Work out the finished part from the listing and answer in its coordinate system (mm). Give positions to 0.01 mm unless a question says otherwise; leave off trailing zeros. Loops run counter-clockwise (first coordinate to the right, second up) from the corner with the lowest first, then second, coordinate; pieces in that order, holes last. Notation, with made-up numbers: M 29.5,35 L 75.5,35 A7 ccw 75.5,40 Z; hole C 15.25,-0.75 d6. An arc over 180 degrees is marked long. Answer in a Markdown table with one row per item. Add a question column.
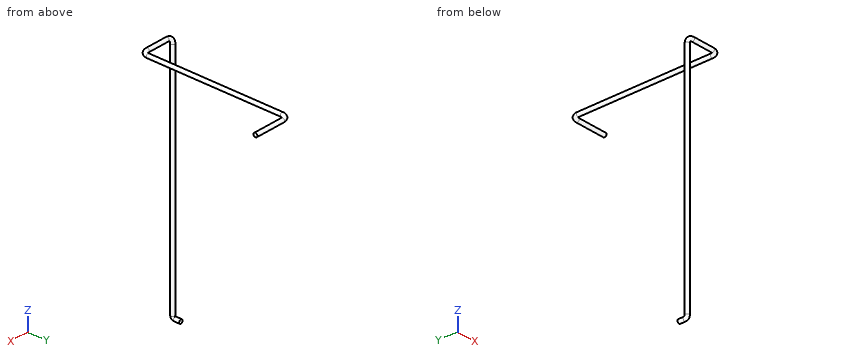
from build123d import *

# Parameters (mm, degrees)
CROQUIS1_R              = 9.525
SALIENTE_EXTRUIR1_DEPTH = 10
CROQUIS2_R              = 9.525


with BuildPart() as part:
    # Croquis1 → Saliente-Extruir1 (new body)
    with BuildSketch(Plane(origin=(0, 0, 0), x_dir=(1, 0, 0), z_dir=(0, 1, 0))):
        with Locations(Location((0, 0, 0), (0, 0, 270))):
            Circle(CROQUIS1_R)
    extrude(amount=-SALIENTE_EXTRUIR1_DEPTH)

    # Barrer1: sweep along a curve in space
    with BuildLine() as barrer1_path:
        Line((0, -10, 0), (0, -28, 0))
        ThreePointArc((0, -28, 0), (0, -36.485281374, 3.514718626), (0, -40, 12))
        Line((0, -40, 12), (0, -40, 1156))
        ThreePointArc((0, -40, 1156), (8.786796564, -40, 1177.213203436), (30, -40, 1186))
        Line((30, -40, 1186), (140, -40, 1186))
        ThreePointArc((140, -40, 1186), (161.213203436, -31.213203436, 1186), (170, -10, 1186))
        Line((170, -10, 1186), (170, 650, 1186))
        ThreePointArc((170, 650, 1186), (178.786796564, 671.213203436, 1186), (200, 680, 1186))
        Line((200, 680, 1186), (350, 680, 1186))
    # Croquis2 → Barrer1 (sweep)
    with BuildSketch(Plane.XZ.offset(10)):
        Circle(CROQUIS2_R)
    sweep(path=barrer1_path.line)


solid = part.part
(1) Consider line 1 along Z through (x, y) = (167, 13.5); line 2 along Z through (x, y) = (177.5, 181). Determine where each line is inside the solid, lowest interval first. Write a range as from..to.
(2) Section A-A, the plane y = 120.5 is taken. Determine the outline of the cut face in (x, z) (3 decimals), and give its area (3 significant figures).
(3) Section B-B, the plane x = 310 is taken. Determine the outline of the cut face in (y, z) (3 decimals).
(4) This flat-tipped pin is pushed along its axis until it touches: P1, Ø5.5, axis at x = 2, z = 1, coming from the +Y side. Where does it stop, or does it pass through?
Numbers:
| question | item | result |
|---|---|---|
| 1 | line 1 | z = 1176.96..1195.04 |
| 1 | line 2 | z = 1180.13..1191.87 |
| 2 | outline | C 170,1186 d19.05 |
| 2 | area | 285 mm² |
| 3 | outline | C 680,1186 d19.05 |
| 4 | P1 | stops at y = 0 |
